```python
from build123d import *

# Parameters (mm, degrees)
SKETCH1_W               = 150
SKETCH1_H               = 45
EXTRUDE1_DEPTH          = 30
CUT_EXTRUDE1_DEPTH      = 29.5
FILLET1_R               = 2
CHAMFER1_SIZE           = 5
SALIENTE_EXTRUIR1_DEPTH = 5


with BuildPart() as part:
    # Sketch1 → Extrude1 (new body)
    with BuildSketch(Plane.XY):
        with Locations((40.803073286, 1.99929078)):
            Rectangle(SKETCH1_W, SKETCH1_H)
    extrude(amount=EXTRUDE1_DEPTH)

    # Sketch2 → Cut-Extrude1 (cut)
    with BuildSketch(Plane.XY.offset(30)):
        Polygon((-34.196926714, 23.99929078), (-34.196926714, -20.00070922), (-33.696926714, -20.00070922), (10.803073286, -20.00070922), (70.803073286, -20.00070922), (115.303073286, -20.00070922), (115.803073286, -20.00070922), (115.803073286, 23.99929078), (115.303073286, 23.99929078), (70.803073286, 23.99929078), (10.803073286, 23.99929078), (-33.696926714, 23.99929078), align=None)
        with BuildLine():
            Line((70.803073286, -19.50070922), (70.803073286, -14.50070922))
            Line((70.803073286, -14.50070922), (73.803073286, -14.50070922))
            ThreePointArc((73.803073286, -14.50070922), (78.752820754, -12.450456688), (80.803073286, -7.50070922))
            Line((80.803073286, -7.50070922), (80.803073286, 11.49929078))
            ThreePointArc((80.803073286, 11.49929078), (78.752820754, 16.449038248), (73.803073286, 18.49929078))
            Line((73.803073286, 18.49929078), (70.803073286, 18.49929078))
            Line((70.803073286, 18.49929078), (70.803073286, 23.49929078))
            Line((70.803073286, 23.49929078), (10.803073286, 23.49929078))
            Line((10.803073286, 23.49929078), (10.803073286, 18.49929078))
            Line((10.803073286, 18.49929078), (7.803073286, 18.49929078))
            ThreePointArc((7.803073286, 18.49929078), (2.853325818, 16.449038248), (0.803073286, 11.49929078))
            Line((0.803073286, 11.49929078), (0.803073286, -7.50070922))
            ThreePointArc((0.803073286, -7.50070922), (2.853325818, -12.450456688), (7.803073286, -14.50070922))
            Line((7.803073286, -14.50070922), (10.803073286, -14.50070922))
            Line((10.803073286, -14.50070922), (10.803073286, -19.50070922))
            Line((10.803073286, -19.50070922), (70.803073286, -19.50070922))
        make_face(mode=Mode.SUBTRACT)
    extrude(amount=-CUT_EXTRUDE1_DEPTH, mode=Mode.SUBTRACT)

    # Fillet1
    fillet1_edges = [part.edges().sort_by_distance(p)[0] for p in [
        (78.752820754, -12.450456688, 30),
        (80.803073286, 1.99929078, 30),
        (78.752820754, 16.449038248, 30),
        (72.303073286, 18.49929078, 30),
        (9.303073286, 18.49929078, 30),
        (2.853325818, 16.449038248, 30),
        (0.803073286, 1.99929078, 30),
        (2.853325818, -12.450456688, 30),
        (9.303073286, -14.50070922, 30),
        (72.303073286, -14.50070922, 30),
    ]]
    fillet(fillet1_edges, radius=FILLET1_R)

    # Chamfer1
    chamfer1_edges = [part.edges().sort_by_distance(p)[0] for p in [
        (40.803073286, 23.49929078, 30),
        (40.803073286, -19.50070922, 30),
    ]]
    chamfer(chamfer1_edges, length=CHAMFER1_SIZE)

    # Croquis1 → Saliente-Extruir1 (add)
    with BuildSketch(Plane(origin=(115.803073286, 0, 0), x_dir=(0, 0, -1), z_dir=(1, 0, 0))):
        Polygon((-0.5, 23.99929078), (-0.5, -20.00070922), (-30, -20.00070922), (-30, -20.50070922), (0, -20.50070922), (0, 24.49929078), (-30, 24.49929078), (-30, 23.99929078), align=None)
    extrude(amount=SALIENTE_EXTRUIR1_DEPTH)


solid = part.part
```
Geometry check sheet. Reference: the model listing, model coordinates, mm. A direction names the side the tool comes from. Round coordinates to 2 decimals unless told otherwise and drop trailing zeros. Order: outer loops, then holes, each group sorted by start corner. A loop starts at its lowest first (then second) coordinate and runs counter-clockwise, first axis right, second up. Notation, with made-up numbers: (37.5, 31) - (70.5, 31) arc R29 ccw to (70.5, 70) - close; hole circle Ø1 at (54, -28.5). An arc over 180 degrees is marked (long way). Use a Markdown table: item, result. Add a question column.
(1) Release check for a two-part mould opening along Y. For faces 4 (the flat face through (42, 2, 0)), 5 (the flat face through (42, 24.499, 15)), 6 (the flat face through (42, -20.001, 15)) record: pulls with the +Y half, pulls with the -Y half, needs draft (parallel to the pull), parting line crosses it, or undercut.
(2) Sectioned sample at A-A, the plane z = 10. Enter the section's corners in (x, y), and give its area (3 significant figures).
(3) Sectioned sample at C-C, the plane y = 10. Enter the section's corners in (x, z).
(4) Tool access check on faces 1 (the flat face through (40.4, -17, 27.5)), 2 (the flat face through (80.803, 2, 14)), 3 (the flat face through (10.803, 21, 15)). Record the directions out of +Z, -Z, +X, -X, +Y, -Y that give a thin tool (end or side, any length) a straight path to the whole face; none if there is none.
(5) Sectioned sample at D-D, the plane x = 98. Enter the section's corners in (y, z), and give its area (3 significant figures).
(6) Depth check by flat-ended pin: pin 1 (5 mm diameter, centred on x = 40.5, y = -6, fed in from -Z); pin 2 (2 mm diameter, centred on y = 20, z = 12.5, fed in from -X); pin 3 (15 mm diameter, centred on y = 2, z = 19.5, fed in from -X); pin 4 (2 mm diameter, centred on y = 21.5, z = 11.5, fed in from +X). Enter the tip coordinate at first touch or a pass-through.
(7) Material ranges on line 1 along Y through (x, z) = (32, 6); line 2 along Y through (x, z) = (104, 28.5); line 3 along Y through (x, z) = (9.5, 25), recorded low to high. Write a range as [from, to].
(8) Sectioned sample at B-B, the plane x = 50. Enter the section's corners in (y, z), and give its area (3 significant figures).
Answers below:
| question | item | result |
|---|---|---|
| 1 | face 4 | needs draft |
| 1 | face 5 | pulls with the +Y half |
| 1 | face 6 | undercut |
| 2 | outline | (-34.2, -20.5) - (120.8, -20.5) - (120.8, -20) - (-34.2, -20) - close; (-34.2, 24) - (120.8, 24) - (120.8, 24.5) - (-34.2, 24.5) - close; (0.8, -7.5) arc R7 ccw to (7.8, -14.5) - (10.8, -14.5) - (10.8, -19.5) - (70.8, -19.5) - (70.8, -14.5) - (73.8, -14.5) arc R7 ccw to (80.8, -7.5) - (80.8, 11.5) arc R7 ccw to (73.8, 18.5) - (70.8, 18.5) - (70.8, 23.5) - (10.8, 23.5) - (10.8, 18.5) - (7.8, 18.5) arc R7 ccw to (0.8, 11.5) - close |
| 2 | area | 3,350 mm² |
| 3 | outline | (-34.2, 0) - (120.8, 0) - (120.8, 0.5) - (80.8, 0.5) - (80.8, 28) arc R2 ccw to (78.8, 30) - (2.8, 30) arc R2 ccw to (0.8, 28) - (0.8, 0.5) - (-34.2, 0.5) - close |
| 4 | face 1 | +Z, +X, -X |
| 4 | face 2 | +Z, +X |
| 4 | face 3 | +Z, -X |
| 5 | outline | (-20.5, 0) - (24.5, 0) - (24.5, 30) - (24, 30) - (24, 0.5) - (-20, 0.5) - (-20, 30) - (-20.5, 30) - close |
| 5 | area | 52.0 mm² |
| 6 | pin 1 | z = 0 |
| 6 | pin 2 | x = 10.8 |
| 6 | pin 3 | x = 0.8 |
| 6 | pin 4 | x = 70.8 |
| 7 | line 1 | [-20.5, -20], [-19.5, 23.5], [24, 24.5] |
| 7 | line 2 | [-20.5, -20], [24, 24.5] |
| 7 | line 3 | [-20.5, -20], [-14.5, 18.5], [24, 24.5] |
| 8 | outline | (-20.5, 0) - (24.5, 0) - (24.5, 30) - (24, 30) - (24, 0.5) - (23.5, 0.5) - (23.5, 25) - (18.5, 30) - (-14.5, 30) - (-19.5, 25) - (-19.5, 0.5) - (-20, 0.5) - (-20, 30) - (-20.5, 30) - close |
| 8 | area | 1,300 mm² |
